Read the model definition and answer for the solid it produces. Units are mm, in the model's axes. A direction names the side the tool comes from. Coordinates: 2 decimals unless noted, no trailing zeros. Write each loop counter-clockwise with the first axis right and the second up, starting at its lowest first coordinate (ties: lowest second). Pieces come first, ordered by that corner, then holes.
(1) Section C-C on y = 9.5 is taken. Write down the section's boundary in (x, z), then the cut area to 3 significant figures.
(2) Section D-D on z = 0 is taken. Write down the section's boundary in (x, y), then the cut area to 3 significant figures.
(3) Section A-A on y = 1.75 is taken. Write down the section's boundary in (x, z), then the cut area to 3 significant figures.
(4) The mould has two halves that part along X. Classify faces 4 (the flat face through (-1, 25, 0)), 5 (the flat face through (50, 12, 0)), 6 (the flat face through (35, 2, 0)): +X half, -X half, draft (parallel to the pull), parting line (faces both ways), or undercut.
(5) Find the intervals of material crossed by probe 1 along X at (y, z) = (10, 0); probe 2 along X at (y, z) = (3.5, 0); probe 3 along X at (y, z) = (3, -4), in increasing order.
(6) Which of the six approach directions +Z, -Z, +X, -X, +Y, -Y give full straight-line access (tool end or side, diameter ignored) to faces 1 (the flat face through (40.7, 0, -1.2)), 2 (the flat face through (-35, 3, 0)), 3 (the flat face through (-42, 15, 0))?
(7) Given pin 1 (2.5 mm diameter, centred on x = 42.5, z = 0, fed in from -Y); pin 2 (3 mm diameter, centred on x = -4.5, z = -1, fed in from -Y), each flat-ended and moving along its own axis, determine where each tip first touches the part or whether it passes through.
(8) Section B-B on x = 42.5 is taken. Write down the section's boundary in (y, z).
from build123d import *

# Parameters (mm, degrees)
BOSS_EXTRU_1_DEPTH      = 25
ENL_V_MAT_EXTRU_1_REACH = 58.789
ESQUISSE3_R             = 2
ENL_V_MAT_EXTRU_2_DEPTH = 15


with BuildPart() as part:
    # Esquisse1 → Boss.-Extru.1 (new body)
    with BuildSketch(Plane(origin=(0, 0, 0), x_dir=(1, 0, 0), z_dir=(0, 1, 0))):
        Polygon((50, 0), (50, 5), (-50, 5), (-50, -5), (50, -5), align=None)
    extrude(amount=BOSS_EXTRU_1_DEPTH)

    # Esquisse2 → Enlèv. mat.-Extru.1 (cut, up to next)
    with BuildSketch(Plane.XY.offset(5), mode=Mode.PRIVATE) as enl_v_mat_extru_1_sk1:
        Polygon((0, 0), (35, 0), (35, 5), (-35, 5), (-35, 0), align=None)
    enl_v_mat_extru_1_tool1 = extrude(enl_v_mat_extru_1_sk1.sketch, amount=-ENL_V_MAT_EXTRU_1_REACH, mode=Mode.PRIVATE) & part.part
    add(enl_v_mat_extru_1_tool1.solids().sort_by_distance((0, 2.5, 5))[0], mode=Mode.SUBTRACT)

    # Esquisse3 → Enlèv. mat.-Extru.2 (cut)
    with BuildSketch(Plane.XZ):
        with Locations(Location((-42.5, 0, 0), (0, 0, 270))):
            Circle(ESQUISSE3_R)
        with Locations(Location((42.5, 0, 0), (0, 0, 270))):
            Circle(ESQUISSE3_R)
    extrude(amount=-ENL_V_MAT_EXTRU_2_DEPTH, mode=Mode.SUBTRACT)


solid = part.part
Response:
1. outline: (-50, -5) - (50, -5) - (50, 5) - (-50, 5) - close; hole circle Ø4 at (-42.5, 0); hole circle Ø4 at (42.5, 0)
1. area: 975 mm2
2. outline: (-50, 0) - (-44.5, 0) - (-44.5, 15) - (-40.5, 15) - (-40.5, 0) - (-35, 0) - (-35, 5) - (35, 5) - (35, 0) - (40.5, 0) - (40.5, 15) - (44.5, 15) - (44.5, 0) - (50, 0) - (50, 25) - (-50, 25) - close
2. area: 2,030 mm2
3. outline: (-50, -5) - (-35, -5) - (-35, 5) - (-50, 5) - close; (35, -5) - (50, -5) - (50, 5) - (35, 5) - close; hole circle Ø4 at (-42.5, 0); hole circle Ø4 at (42.5, 0)
3. area: 275 mm2
4. face 4: draft
4. face 5: +X half
4. face 6: undercut
5. probe 1: x = -50 to -44.5, -40.5 to 40.5, 44.5 to 50
5. probe 2: x = -50 to -44.5, -40.5 to -35, 35 to 40.5, 44.5 to 50
5. probe 3: x = -50 to -35, 35 to 50
6. face 1: +Z, -Z, +X, -X, -Y
6. face 2: +Z, -Z, -Y
6. face 3: -Y
7. pin 1: stops at y = 15
7. pin 2: stops at y = 5
8. outline: (0, -5) - (25, -5) - (25, 5) - (0, 5) - (0, 2) - (15, 2) - (15, -2) - (0, -2) - close
